Could you check a few things on this model? Use its own coordinates, in mm. A direction names the side the tool comes from. Round coordinates to 2 decimals unless told otherwise and drop trailing zeros. Write each loop counter-clockwise with the first axis right and the second up, starting at its lowest first coordinate (ties: lowest second). Pieces come first, ordered by that corner, then holes. Notation, with made-up numbers: (87, -19.75) -> (131, -19.75) arc R19 ccw to (131, 2.25) -> close; hole circle Ø7 at (59.5, -19.75). An arc over 180 degrees is marked (long way). One line per question, with ' | ' between items. Start each with the question number.
1. Imagine slicing it at B-B, the plane y = 9. List the corners of the cut face in (x, z) for me.
2. If I drill on line 1 along X through (y, z) = (30, 9); line 2 along X through (y, z) = (0.5, 0.5); line 3 along X through (y, z) = (41.5, 3.25), over which ranges is the centre line in solid material (lowest first)? Write a range as [from, to].
3. Thinking about a two-plate mould opening in X: for faces 4 (the cylindrical face through (29.42, 27.13, 4.82)), 5 (the cylindrical face through (1, 45.49, 4.68)), 6 (the flat face through (-45, 0, 5)), which applies, released by +X, released by -X, zero draft, split by the parting line, or undercut?
4. Imagine slicing it at D-D, the plane y = 43.5. List the corners of the cut face in (x, z) for me.
5. For faces 1 (the cylindrical face through (39.15, -1.03, 4.82)), 2 (the flat face through (36, 0, 5)), 3 (the flat face through (45, 0, 5)), which set-ups out of +Z, -Z, +X, -X, +Y, -Y let a thin tool reach every point of the face, with its end or its side?
6. Imagine slicing it at A-A, the plane x = 0. List the corners of the cut face in (y, z) for me, and give its area (3 significant figures).
7. Imagine slicing it at C-C, the plane z = 5. List the corners of the cut face in (x, y) for me, and give its area (3 significant figures).
8. For pin 1 Ø0.5 at (x, z) = (-44.5, 6.5) entering from -Y; pin 2 Ø4 at (x, z) = (33.5, 3) entering from +Y; pin 3 Ø2 at (y, z) = (18, 3.5) entering from -X, each with a flat end and sliding along its axis, tell me the tip position at first contact or that it passes through.
from build123d import *

# Parameters (mm, degrees)
SALIENTE_EXTRUIR1_DEPTH = 9.5
CROQUIS2_R              = 1.7
CORTAR_EXTRUIR1_DEPTH   = 10.5
CROQUIS3_R              = 3.4
CROQUIS3_R_2            = 1.7
SALIENTE_EXTRUIR2_DEPTH = 9.5


with BuildPart() as part:
    # Croquis1 → Saliente-Extruir1 (new body)
    with BuildSketch(Plane.XY):
        with BuildLine():
            Line((-45.5, 0), (-35.5, 0))
            ThreePointArc((-35.5, 0), (0, 35.5), (35.5, 0))
            Line((35.5, 0), (45.5, 0))
            ThreePointArc((45.5, 0), (0, 45.5), (-45.5, 0))
        make_face()
    extrude(amount=SALIENTE_EXTRUIR1_DEPTH)

    # Croquis2 → Cortar-Extruir1 (cut, through all)
    with BuildSketch(Plane.XY.offset(9.5)):
        with Locations((0, 40.5)):
            Circle(CROQUIS2_R)
        with Locations((28.637824638, 28.637824638)):
            Circle(CROQUIS2_R)
        with Locations((40.5, 0)):
            Circle(CROQUIS2_R)
        with Locations((-40.5, 0)):
            Circle(CROQUIS2_R)
        with Locations((-28.637824638, 28.637824638)):
            Circle(CROQUIS2_R)
    extrude(amount=-CORTAR_EXTRUIR1_DEPTH, mode=Mode.SUBTRACT)

    # Croquis3 → Saliente-Extruir2 (add)
    with BuildSketch(Plane.XY.offset(9.5)):
        with Locations((-40.5, 0)):
            Circle(CROQUIS3_R)
        with Locations((-40.5, 0)):
            Circle(CROQUIS3_R_2, mode=Mode.SUBTRACT)
        with Locations((40.5, 0)):
            Circle(CROQUIS3_R)
        with Locations((40.5, 0)):
            Circle(CROQUIS3_R_2, mode=Mode.SUBTRACT)
    extrude(amount=-SALIENTE_EXTRUIR2_DEPTH)


solid = part.part
Geometry results:
1) outline: (-44.6, 0) -> (-34.34, 0) -> (-34.34, 9.5) -> (-44.6, 9.5) -> close; (34.34, 0) -> (44.6, 0) -> (44.6, 9.5) -> (34.34, 9.5) -> close
2) line 1: x = [-34.21, -29.65], [-27.62, -18.98], [18.98, 27.62], [29.65, 34.21] | line 2: x = [-45.5, -42.12], [-38.88, -35.5], [35.5, 38.88], [42.12, 45.5] | line 3: x = [-18.65, -1.37], [1.37, 18.65]
3) face 4: undercut | face 5: split by the parting line | face 6: zero draft
4) outline: (-13.34, 0) -> (13.34, 0) -> (13.34, 9.5) -> (-13.34, 9.5) -> close
5) face 1: +Z, -Z | face 2: +Z, -Z, -Y | face 3: +Z, -Z, +X, -Y
6) outline: (35.5, 0) -> (38.8, 0) -> (38.8, 9.5) -> (35.5, 9.5) -> close; (42.2, 0) -> (45.5, 0) -> (45.5, 9.5) -> (42.2, 9.5) -> close | area: 62.7 mm2
7) outline: (-45.5, 0) -> (-43.9, 0) arc R3.4 ccw to (-37.1, 0) -> (-35.5, 0) arc R35.5 cw to (35.5, 0) -> (37.1, 0) arc R3.4 ccw to (43.9, 0) -> (45.5, 0) arc R45.5 ccw to start; hole circle Ø3.4 at (-40.5, 0); hole circle Ø3.4 at (-28.64, 28.64); hole circle Ø3.4 at (0, 40.5); hole circle Ø3.4 at (28.64, 28.64); hole circle Ø3.4 at (40.5, 0) | area: 1,260 mm2
8) pin 1: stops at y = 0 | pin 2: stops at y = 32.83 | pin 3: stops at x = -42.2
